Autodesk Fusion 360 part; units mm, degrees
sketch "Skizze1" plane through (0, 0, 0) normal (0, 0, 1) x (1, 0, 0)
  line L0 (0, 80) -> (0, -42.0959) construction
  line L1 (-31.8813, 0) -> (31.8813, 0)
  line L2 (31.8813, 0) -> (31.8813, 3)
  line L3 (-31.8813, 3) -> (-31.8813, 0)
  line L4 (-26.4649, 3) -> (-19.1093, 10.3556)
  line L5 (26.4649, 3) -> (18.216, 9.5813)
  line L6 (-42, 31.5) -> (42, 31.5) construction
  arc A0 (-23.5276, 40.3158) -> (23.5276, 40.3158) centre (0, 31.5) ccw
  line L7 (23.5276, 40.3158) -> (26.688, 41.5)
  line L8 (-23.5276, 40.3158) -> (-26.688, 41.5)
  arc A1 (18.216, 9.5813) -> (26.688, 41.5) centre (0, 31.5) ccw
  arc A2 (-26.688, 41.5) -> (-19.1093, 10.3556) centre (0, 31.5) ccw
  line L9 (-23.5276, 40.3158) -> (0, 31.5) construction
  line L10 (0, 31.5) -> (23.5276, 40.3158) construction
  line L11 (31.8813, 3) -> (26.4649, 3)
  line L12 (-26.4649, 3) -> (-31.8813, 3)
  arc A3 (-19.1093, 10.3556) -> (18.216, 9.5813) centre (0, 31.5) ccw
  line L13 (-26.4649, 3) -> (26.4649, 3)
  dimension "d1" = 50.25
  dimension "d2" = 3
  dimension "d4" = 31.5
  dimension "d5" = 135
  dimension "d6" = 10
extrude "Extrusion1" add sketch "Skizze1" along normal blind 8
fillet "Abrundung1" radius 1 4 edges at (-23.5276, 40.3158, 4) (-26.688, 41.5, 4) (26.688, 41.5, 4) (23.5276, 40.3158, 4)
sketch "Skizze2" plane through (0, 0, 8) normal (0, 0, 1) x (-1, 0, 0)
  arc A0 (-24.4461, -40.6599) -> (-23.8478, -39.4088) centre (-24.797, -39.7235) ccw
  arc A1 (23.8478, -39.4088) -> (-23.8478, -39.4088) centre (0, -31.5) ccw
  arc A2 (23.8478, -39.4088) -> (24.4461, -40.6599) centre (24.797, -39.7235) ccw
  line L0 (24.4461, -40.6599) -> (25.7346, -41.1427)
  arc A3 (25.7346, -41.1427) -> (27.034, -40.5229) centre (26.0854, -40.2063) ccw
  arc A4 (27.034, -40.5229) -> (19.1093, -10.3556) centre (0, -31.5) ccw
  line L1 (19.1093, -10.3556) -> (26.4649, -3)
  line L2 (26.4649, -3) -> (31.8813, -3)
  line L3 (31.8813, -3) -> (31.8813, 0)
  line L4 (31.8813, 0) -> (-31.8813, 0)
  line L5 (-31.8813, 0) -> (-31.8813, -3)
  line L6 (-31.8813, -3) -> (-26.4649, -3)
  line L7 (-26.4649, -3) -> (-18.216, -9.5813)
  arc A5 (-18.216, -9.5813) -> (-27.034, -40.5229) centre (0, -31.5) ccw
  arc A6 (-27.034, -40.5229) -> (-25.7346, -41.1427) centre (-26.0854, -40.2063) ccw
  line L8 (-25.7346, -41.1427) -> (-24.4461, -40.6599)
  arc A7 (23.8478, -39.4088) -> (-23.8478, -39.4088) centre (0, -31.5) ccw
  arc A8 (27.034, -40.5229) -> (19.1093, -10.3556) centre (0, -31.5) ccw
  arc A9 (-18.216, -9.5813) -> (-27.034, -40.5229) centre (0, -31.5) ccw
  line L9 (31.8813, 0) -> (-31.8813, 0)
  circle A10 centre (0, -31.5) radius 28.5
  line L10 (16.7677, -8.4546) -> (22.2223, -3)
  line L11 (-15.725, -7.7308) -> (-21.6546, -3)
  line L12 (22.2223, -3) -> (-26.4649, -3)
  line L13 (12.9109, -3) -> (10.7896, -5.1213)
  line L14 (-12.5011, -3) -> (-10.1561, -4.871)
  dimension "d13" = 3
  dimension "d14" = 3
  dimension "d15" = 3
  dimension "d16" = 3
extrude "Extrusion2" cut sketch "Skizze2" against normal up to surface (8 mm away) contours A10 L11 L12 L14 | A10 L10 L12 L13
fillet "Abrundung2" radius 3 2 edges at (-19.1093, 10.3556, 4) (18.216, 9.5813, 4)
fillet "Abrundung3" radius 1.5 4 edges at (31.8813, 3, 4) (26.4649, 3, 4) (-26.4649, 3, 4) (-31.8813, 3, 4)
fillet "Abrundung4" radius 1 4 edges at (21.6546, 3, 4) (15.725, 7.7308, 4) (10.1561, 4.871, 4) (12.5011, 3, 4)
fillet "Abrundung5" radius 1 4 edges at (-12.9109, 3, 4) (-10.7896, 5.1213, 4) (-16.7677, 8.4546, 4) (-22.2223, 3, 4)
sketch "Skizze3" plane through (0, 0, 0) normal (0, -1, 0) x (1, 0, 0)
  line L0 (-31.8813, 0) -> (31.8813, 0)
  line L1 (31.8813, 0) -> (31.8813, 8)
  line L2 (31.8813, 8) -> (-31.8813, 8)
  line L3 (-31.8813, 8) -> (-31.8813, 0)
equation "d4 = ( 63 / 2 ) * 1 mm"
CAD build for the part. Positions are in the model's coordinates, mm. A direction names the side the tool comes from. Round coordinates to 2 decimals unless told otherwise and drop trailing zeros. Write each loop counter-clockwise with the first axis right and the second up, starting at its lowest first coordinate (ties: lowest second). Pieces come first, ordered by that corner, then holes. Notation, with made-up numbers: M -25.5,56 L -13.5,56 A23 cw -13.5,91 Z; hole C 68.25,-14 d5. An arc over 180 degrees is marked long. Put each result on its own line as item: value. Start each with the question number.
1) Saw through at B-B, the plane x = -18. Write the cut outline in (y, z).
2) Saw through at D-D, the plane z = 6. Count the separate pieces of the cut face and the enclosed holes in it, and give its area (3 significant figures).
3) Saw through at A-A, the plane y = 31.5. Write the cut outline in (x, z).
4) Pin check, flat tips, straight feed: pin 1 Ø3 at (x, z) = (17, 6) entering from +Y; pin 2 Ø1.9 at (x, z) = (-15, 3.5) entering from +Y; pin 3 Ø3 at (x, y) = (-24.5, 28) entering from -Z; pin 4 Ø1 at (x, z) = (16, 3) entering from +Y. Stop position of each tip, or through.
5) Pull direction X, two halves, no side cores. Call faces 6 (the flat face through (-23.661, 5.804, 3.944)), 7 (the flat face through (-29, 3, 4)), 8 (the flat face through (-17, 3, 4)): pulls with the +X half, pulls with the -X half, needs draft (parallel to the pull), parting line crosses it, or undercut.
6) Saw through at C-C, the plane x = 0. Write the cut outline in (y, z), and give its area (3 significant figures).
7) Drill centre lines: probe 1 along X at (y, z) = (3.5, 7); probe 2 along X at (y, z) = (31.5, 3.75); probe 3 along X at (y, z) = (6, 6.75). Where is each one in solid material? Low to high. Write a range as [from, to].
8) 3-axis set-ups, long thin cutter, end or side, ignore diameter. For faces 1 (the cylindrical face through (-27.85, 25.44, 3.94)), 2 (the cylindrical face through (-31.4, 2.6, 4.1)), 3 (the flat face through (23.53, 5.34, 3.94)), 4 (the flat face through (17.83, 6.05, 4.06)), 5 (the flat face through (-25.081, 40.898, 3.944)): which of +Z, -Z, +X, -X, +Y, -Y reach the whole face in a straight line?
Resolved:
1. outline: M 0,0 L 3,0 L 3,8 L 0,8 Z; M 7.22,0 L 13.97,0 L 13.97,8 L 7.22,8 Z
2. separate pieces: 1
2. enclosed holes: 2
2. area: 620 mm²
3. outline: M -28.5,0 L -25.13,0 L -25.13,8 L -28.5,8 Z; M 25.13,0 L 28.5,0 L 28.5,8 L 25.13,8 Z
4. pin 1: y = 14.5
4. pin 2: y = 12.09
4. pin 3: z = 0
4. pin 4: y = 12.55
5. face 6: pulls with the -X half
5. face 7: needs draft
5. face 8: undercut
6. outline: M 0,0 L 6.37,0 L 6.37,8 L 0,8 Z
6. area: 51.0 mm²
7. probe 1: [-25.96, -20.67], [-12.41, 11.87], [19.66, 25.84]
7. probe 2: [-28.5, -25.13], [25.13, 28.5]
7. probe 3: [-23.46, -19.22], [-12.73, 12.73], [17.89, 22.7]
8. face 1: +Z, -Z, -X
8. face 2: +Z, -Z, -X, +Y
8. face 3: +Z, -Z, +X
8. face 4: +Z, -Z
8. face 5: +Z, -Z, +Y
